Model file for the job. Use its own axes, mm. Face numbers are marked on the shaded views. A direction names the side the tool comes from. Give positions to 0.01 mm unless a question says otherwise; leave off trailing zeros. Order: outer loops, then holes, each group sorted by start corner. A loop starts at its lowest first (then second) coordinate and runs counter-clockwise, first axis right, second up. Notation, with made-up numbers: (80, 6.5) -> (129, 6.5) arc R17 ccw to (129, 34.5) -> close; hole circle Ø1 at (19.25, -17.5). An arc over 180 degrees is marked (long way). Use CSV: the item, a comma, the result in double quotes. Start each with the question number.
1. 3-axis set-ups, long thin cutter, end or side, ignore diameter. For the marked faces 1, 2, 3, 4 and 5: which of +Z, -Z, +X, -X, +Y, -Y reach the whole face in a straight line?
2. Drop flat-ended pins along their axis: pin 1 (2 mm diameter, centred on x = 71, y = -19.5, fed in from -Z); pin 2 (4 mm diameter, centred on x = 77, y = -9, fed in from +Z); pin 3 (11 mm diameter, centred on y = -18.5, z = -2, fed in from +X). Give the stop position or say it passes through.
3. Cut at A-A on x = 71. List the corners of the cut face in (y, z).
4. Cut at B-B on x = 31. List the corners of the cut face in (y, z), then the cut area to 3 significant figures.
5. Pull direction X, two halves, no side cores. Call the marked faces 6, 7 and 8: released by +X, released by -X, zero draft, split by the parting line, or undercut.
6. Wall check: line 1 (Z direction, x = 97, y = -22) (3 decimals); line 2 (Y direction, x = 99, z = 0); line 3 (Y direction, x = 97.75, z = 0) (3 decimals). Give the ranges that are in metal, low to high. Write a range as from..to.
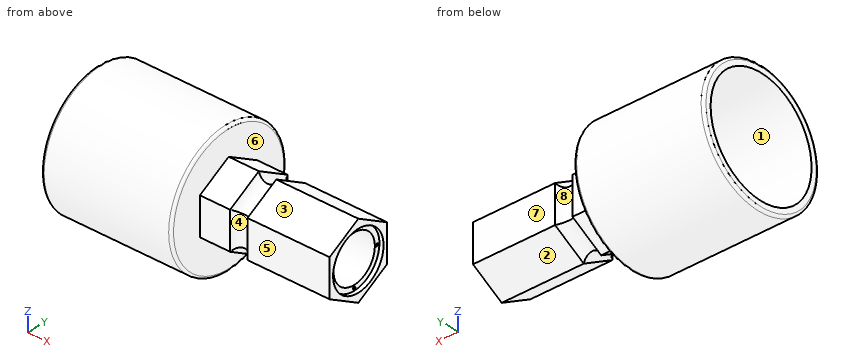
```python
from build123d import *

# Parameters (mm, degrees)
BOSS_EXTRUDE3_DEPTH = 50
BOSS_EXTRUDE4_START = -53
SKETCH6_R           = 12.5
SKETCH6_R_2         = 9
BOSS_EXTRUDE4_DEPTH = 53
SKETCH3_W           = 3.5
SKETCH3_H           = 14.43375673
CIRPATTERN4_COUNT   = 6
FILLET1_R           = 1
SKETCH8_R           = 11
CUT_EXTRUDE1_DEPTH  = 1.6
CIRPATTERN5_COUNT   = 4


with BuildPart() as part:
    # Sketch1 → Revolve1 (revolve)
    with BuildSketch(Plane.XY):
        with BuildLine():
            ThreePointArc((0, 2), (0.292893219, 2.707106781), (1, 3))
            Line((1, 3), (49, 3))
            ThreePointArc((49, 3), (49.707106781, 2.707106781), (50, 2))
            Line((50, 2), (50, -12))
            Line((50, -12), (48, -12))
            ThreePointArc((48, -12), (47.292893219, -11.707106781), (47, -11))
            Line((47, -11), (47, -1))
            ThreePointArc((47, -1), (46.707106781, -0.292893219), (46, 0))
            Line((46, 0), (0, 0))
            Line((0, 0), (0, 2))
        make_face()
    revolve(axis=Axis((50, -22, 0), (-1, 0, 0)))

    # Sketch2 → Boss-Extrude3 (add)
    with BuildSketch(Plane(origin=(50, 0, 0), x_dir=(0, 0, -1), z_dir=(1, 0, 0))):
        Polygon((14.43375673, -22), (7.216878365, -9.5), (-7.216878365, -9.5), (-14.43375673, -22), (-7.216878365, -34.5), (7.216878365, -34.5), align=None)
        Polygon((11.547005384, -22), (5.773502692, -12), (-5.773502692, -12), (-11.547005384, -22), (-5.773502692, -32), (5.773502692, -32), align=None, mode=Mode.SUBTRACT)
    extrude(amount=BOSS_EXTRUDE3_DEPTH)

    # Sketch6 → Boss-Extrude4 (add)
    with BuildSketch(Plane.ZY.offset(-47).offset(BOSS_EXTRUDE4_START)):
        with Locations((0, -22)):
            Circle(SKETCH6_R)
        with Locations(Location((0, -22, 0), (0, 0, 270))):
            Circle(SKETCH6_R_2, mode=Mode.SUBTRACT)
    extrude(amount=BOSS_EXTRUDE4_DEPTH)

    # Sketch3 → Cut-Revolve3 (revolve, cut)
    with BuildSketch(Plane(origin=(0, -8.5, 0), x_dir=(1, 0, 0), z_dir=(0, 1, 0))):
        with Locations((66.75, 0)):
            Rectangle(SKETCH3_W, SKETCH3_H)
    cut_revolve3 = revolve(axis=Axis((65, -8.5, -7.216878365), (0, 0, 1)), mode=Mode.SUBTRACT)

    # CirPattern4: Cut-Revolve3 ×6 about axis
    cirpattern4_axis = Axis((0, -22, 0), (-1, 0, 0))
    for i in range(1, CIRPATTERN4_COUNT):
        add(cut_revolve3.rotate(cirpattern4_axis, i * 360 / CIRPATTERN4_COUNT), mode=Mode.SUBTRACT)

    # Fillet1
    fillet1_edges = [part.edges().sort_by_distance(p)[0] for p in [
        (47, -13, 0),
    ]]
    fillet(fillet1_edges, radius=FILLET1_R)

    # Sketch8 → Cut-Extrude1 (cut)
    with BuildSketch(Plane(origin=(100, 0, 0), x_dir=(0, 0, -1), z_dir=(1, 0, 0))):
        with Locations((0, -22)):
            Circle(SKETCH8_R)
    extrude(amount=-CUT_EXTRUDE1_DEPTH, mode=Mode.SUBTRACT)

    # Sketch10 → Tap Drill for M1.2x0.25 Tap1 (revolve, cut)
    with BuildSketch(Plane(origin=(98.4, -12, 0), x_dir=(0, 0, -1), z_dir=(0, 1, 0))):
        Polygon((0, 0), (0, 2.285408794), (0.475, 2), (0.475, 0.025), (0.5, 0), align=None)
    tap_drill_for_m1_2x0_25_tap1 = revolve(axis=Axis((104.75, -12, 0), (-1, 0, 0)), mode=Mode.SUBTRACT)

    # CirPattern5: Tap Drill for M1.2x0.25 Tap1 ×4 about axis
    cirpattern5_axis = Axis((0, -22, 0), (1, 0, 0))
    for i in range(1, CIRPATTERN5_COUNT):
        add(tap_drill_for_m1_2x0_25_tap1.rotate(cirpattern5_axis, i * 360 / CIRPATTERN5_COUNT), mode=Mode.SUBTRACT)


solid = part.part
```
Verdict:
1,face 1,"-X"
1,face 2,"-Z, +X, +Y"
1,face 3,"+Z, +X, -Y"
1,face 4,"+Z, -Z, -Y"
1,face 5,"+Z, -Z, +X, -Y"
2,pin 1,"z = -13.57"
2,pin 2,"z = 8.08"
2,pin 3,"x = 98.4"
3,outline,"(-34.5, -7.22) -> (-22, -14.43) -> (-9.5, -7.22) -> (-9.5, 7.22) -> (-22, 14.43) -> (-34.5, 7.22) -> close; hole circle Ø18 at (-22, 0)"
4,outline,"circle Ø50 at (-22, 0); hole circle Ø44 at (-22, 0)"
4,area,"443 mm^2"
5,face 6,"released by +X"
5,face 7,"zero draft"
5,face 8,"undercut"
6,line 1,"-14.434..-10.475, -9.525..-9, 9..9.525, 10.475..14.434"
6,line 2,"-34.5..-33, -11..-9.5"
6,line 3,"-34.5..-32.475, -31.525..-31, -13..-12.475, -11.525..-9.5"
